Input: part model. Units: mm. Frame: model coordinates. A direction names the side the tool comes from. Coordinates: 2 decimals unless noted, no trailing zeros. Order: outer loops, then holes, each group sorted by start corner. A loop starts at its lowest first (then second) coordinate and runs counter-clockwise, first axis right, second up. Notation, with made-up numbers: (86.25, 7.5) - (138.25, 7.5) arc R21 ccw to (138.25, 33.5) - close; hole circle Ø1 at (59.5, -27.5). An arc over 180 degrees is marked (long way). Answer as CSV lines item,"result". Start each with the question number.
Item 1: First-contact query: pin 1 (5 mm diameter, centred on x = -10.5, z = -3.5, fed in from -Y); pin 2 (2 mm diameter, centred on x = -7, y = 1.5, fed in from +Z); pin 3 (2 mm diameter, centred on x = -5.5, y = 3.5, fed in from +Z); pin 4 (1 mm diameter, centred on y = -5.5, z = -6, fed in from +X). Flat tips, straight axial feed; report the tip coordinate or a pass-through.
Item 2: Access query for faces 5 (the cylindrical face through (-0.175, -7.493, -0.33)), 6 (the cylindrical face through (-13.06, -0.93, -7.09)). Directions: +Z, -Z, +X, -X, +Y, -Y. A direction counts if a zero-diameter tool reaches every point of the face in a straight line with its end or side. Return the directions, or none.
Item 3: Section A-A (z = 0). Output: boundary loops of the cut face in (x, y).
Item 4: Draft query along X for faces 1 (the cylindrical face through (15.818, -7.493, -0.33)), 2 (the flat face through (-18.5, 3, 3)), 3 (the cylindrical face through (13.04, -0.93, -7.09)), 4 (the flat face through (18.5, -3, 3)). Return one class per face: +X half, -X half, draft (parallel to the pull), parting line (faces both ways), or undercut.
Item 5: Section C-C (x = -15). Output: boundary loops of the cut face in (y, z).
Item 6: Material intervals for line 1 along Y through (x, z) = (-9, 0); line 2 along X through (y, z) = (-4, -6), sorted ascending.
from build123d import *


with BuildPart() as part:
    # Sketch1 → Revolve1 (revolve)
    with BuildSketch(Plane.XY):
        with BuildLine():
            Line((-18.5, 7.1), (-18.5, 4))
            Line((-18.5, 4), (18.5, 4))
            Line((18.5, 4), (18.5, 7.1))
            ThreePointArc((18.5, 7.1), (18.382842712, 7.382842712), (18.1, 7.5))
            Line((18.1, 7.5), (13.6, 7.5))
            Line((13.6, 7.5), (13.6, 7.15))
            Line((13.6, 7.15), (12.5, 7.15))
            Line((12.5, 7.15), (12.5, 7.5))
            Line((12.5, 7.5), (-12.5, 7.5))
            Line((-12.5, 7.5), (-12.5, 7.15))
            Line((-12.5, 7.15), (-13.6, 7.15))
            Line((-13.6, 7.15), (-13.6, 7.5))
            Line((-13.6, 7.5), (-18.1, 7.5))
            ThreePointArc((-18.1, 7.5), (-18.382842712, 7.382842712), (-18.5, 7.1))
        make_face()
    revolve(axis=Axis((18.5, 0, 0), (-1, 0, 0)))


solid = part.part
Determined:
1,pin 1,"stops at y = -7.43"
1,pin 2,"stops at z = 7.48"
1,pin 3,"stops at z = 7.07"
1,pin 4,"passes through"
2,face 5,"+X, -X"
2,face 6,"none"
3,outline,"(-18.5, -7.1) arc R0.4 ccw to (-18.1, -7.5) - (-13.6, -7.5) - (-13.6, -7.15) - (-12.5, -7.15) - (-12.5, -7.5) - (12.5, -7.5) - (12.5, -7.15) - (13.6, -7.15) - (13.6, -7.5) - (18.1, -7.5) arc R0.4 ccw to (18.5, -7.1) - (18.5, -4) - (-18.5, -4) - close; (-18.5, 4) - (18.5, 4) - (18.5, 7.1) arc R0.4 ccw to (18.1, 7.5) - (13.6, 7.5) - (13.6, 7.15) - (12.5, 7.15) - (12.5, 7.5) - (-12.5, 7.5) - (-12.5, 7.15) - (-13.6, 7.15) - (-13.6, 7.5) - (-18.1, 7.5) arc R0.4 ccw to (-18.5, 7.1) - close"
4,face 1,"draft"
4,face 2,"-X half"
4,face 3,"undercut"
4,face 4,"+X half"
5,outline,"circle Ø15 at (0, 0); hole circle Ø8 at (0, 0)"
6,line 1,"y = -7.5 to -4, 4 to 7.5"
6,line 2,"x = -18.48 to -13.6, -12.5 to 12.5, 13.6 to 18.48"
